```python
from build123d import *

# Parameters (mm, degrees)
SKETCH1_W           = 24
SKETCH1_H           = 11.708497378
SKETCH1_R           = 1.5
BOSS_EXTRUDE1_DEPTH = 2
CHAMFER1_SIZE       = 2


with BuildPart() as part:
    # Sketch1 → Boss-Extrude1 (new body)
    with BuildSketch(Plane.XY):
        Rectangle(SKETCH1_W, SKETCH1_H)
        with Locations((-9, 0)):
            Circle(SKETCH1_R, mode=Mode.SUBTRACT)
        with Locations((-4, 0)):
            Circle(SKETCH1_R, mode=Mode.SUBTRACT)
        with Locations(Location((4, 0, 0), (0, 0, 180))):
            Circle(SKETCH1_R, mode=Mode.SUBTRACT)
        with Locations(Location((9, 0, 0), (0, 0, 180))):
            Circle(SKETCH1_R, mode=Mode.SUBTRACT)
    extrude(amount=BOSS_EXTRUDE1_DEPTH)

    # Chamfer1
    chamfer1_edges = [part.edges().sort_by_distance(p)[0] for p in [
        (12, -5.854248689, 1),
        (-12, -5.854248689, 1),
        (-12, 5.854248689, 1),
        (12, 5.854248689, 1),
    ]]
    chamfer(chamfer1_edges, length=CHAMFER1_SIZE)


solid = part.part
```
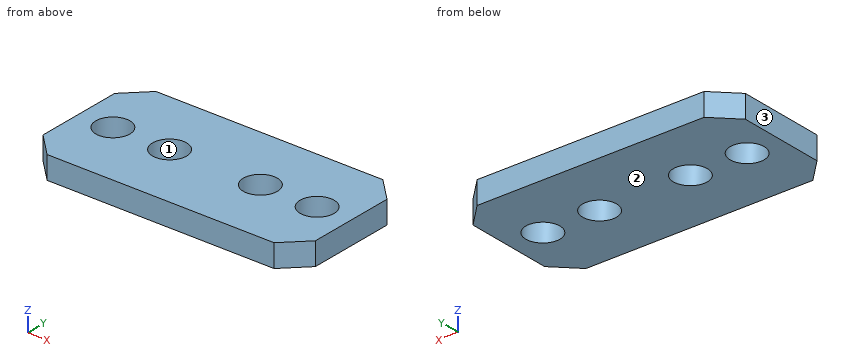
Check sheet for the modelled part. Datum: model origin and axes. Units: mm. Face numbers are marked on the shaded views. Give positions to 0.01 mm unless a question says otherwise; leave off trailing zeros. Write each loop counter-clockwise with the first axis right and the second up, starting at its lowest first coordinate (ties: lowest second). Pieces come first, ordered by that corner, then holes. Notation, with made-up numbers: (-31, -7) -> (5, -7) arc R33 cw to (5, 23) -> close; hole circle Ø3 at (-26, 16). An arc over 180 degrees is marked (long way). Use CSV: the item, a comma, the result in double quotes. Start each with the question number.
Q1. Cross-section at C-C on z = 1.65. Enter the section's corners in (x, y).
Q2. Release check for a two-part mould opening along X. For the marked faces 1, 2 and 3 record: +X half, -X half, draft (parallel to the pull), parting line (faces both ways), or undercut.
Q3. Cross-section at D-D on x = -3.5. Enter the section's corners in (y, z), and give its area (3 significant figures).
Q4. Cross-section at A-A on x = -9. Enter the section's corners in (y, z).
Q5. Cross-section at B-B on y = 0. Enter the section's corners in (x, z), and give its area (3 significant figures).
Q6. Scan lines: line 1 along Y through (x, z) = (9, 1.2); line 2 along X through (y, z) = (-1.25, 0.85); line 3 along Y through (x, z) = (-4.5, 1.1). Record each from-to range of solid material in increasing order.
Q7. Depth check by flat-ended pin: P1, Ø1.8, axis at x = 9, y = 0, coming from the -Z side. Enter the tip coordinate at first touch or a pass-through.
Working result:
1,outline,"(-12, -3.85) -> (-10, -5.85) -> (10, -5.85) -> (12, -3.85) -> (12, 3.85) -> (10, 5.85) -> (-10, 5.85) -> (-12, 3.85) -> close; hole circle Ø3 at (-9, 0); hole circle Ø3 at (-4, 0); hole circle Ø3 at (4, 0); hole circle Ø3 at (9, 0)"
2,face 1,"undercut"
2,face 2,"draft"
2,face 3,"-X half"
3,outline,"(-5.85, 0) -> (-1.41, 0) -> (-1.41, 2) -> (-5.85, 2) -> close; (1.41, 0) -> (5.85, 0) -> (5.85, 2) -> (1.41, 2) -> close"
3,area,"17.8 mm^2"
4,outline,"(-5.85, 0) -> (-1.5, 0) -> (-1.5, 2) -> (-5.85, 2) -> close; (1.5, 0) -> (5.85, 0) -> (5.85, 2) -> (1.5, 2) -> close"
5,outline,"(-12, 0) -> (-10.5, 0) -> (-10.5, 2) -> (-12, 2) -> close; (-7.5, 0) -> (-5.5, 0) -> (-5.5, 2) -> (-7.5, 2) -> close; (-2.5, 0) -> (2.5, 0) -> (2.5, 2) -> (-2.5, 2) -> close; (5.5, 0) -> (7.5, 0) -> (7.5, 2) -> (5.5, 2) -> close; (10.5, 0) -> (12, 0) -> (12, 2) -> (10.5, 2) -> close"
5,area,"24.0 mm^2"
6,line 1,"y = -5.85 to -1.5, 1.5 to 5.85"
6,line 2,"x = -12 to -9.83, -8.17 to -4.83, -3.17 to 3.17, 4.83 to 8.17, 9.83 to 12"
6,line 3,"y = -5.85 to -1.41, 1.41 to 5.85"
7,P1,"passes through"
